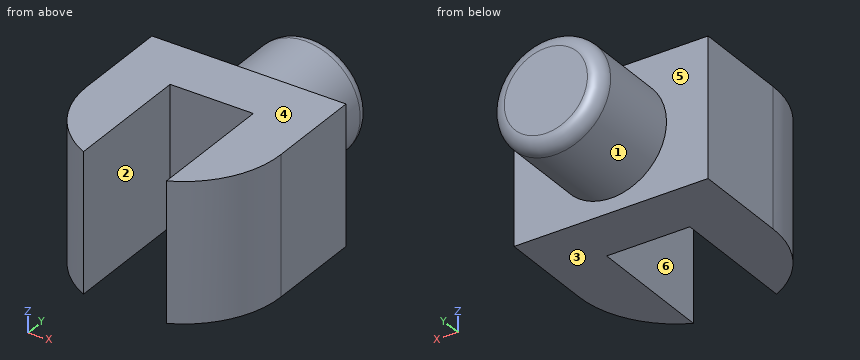
from build123d import *

# Parameters (mm, degrees)
HAND_DEPTH            = 2.5
HAND_DEPTH_BACK       = 2.5
SKETCH3_R             = 2
WRIST_DEPTH           = 7
FINGER_GAP_DEPTH      = 1.5
FINGER_GAP_DEPTH_BACK = 9.215838363
SKETCH2_W             = 3
SKETCH2_H             = 6
EASY_INSERT_R         = 0.5
SCALE1_SCALE          = 2


with BuildPart() as part:
    # Sketch1 → Hand (new, two sides: drawn at the far end of the back side and taken through both)
    with BuildSketch(Plane.XY.offset(-HAND_DEPTH_BACK)):
        with BuildLine():
            Line((-3.5, 0), (-3.5, 3.5))
            Line((-3.5, 3.5), (3.5, 3.5))
            Line((3.5, 3.5), (3.5, 0))
            ThreePointArc((3.5, 0), (0, -3.5), (-3.5, 0))
        make_face()
    extrude(amount=HAND_DEPTH + HAND_DEPTH_BACK)

    # Sketch3 → Wrist (add)
    with BuildSketch(Plane(origin=(0, 0, 0), x_dir=(1, 0, 0), z_dir=(0, 1, 0))):
        with Locations(Location((0, 0, 0), (0, 0, 270))):
            Circle(SKETCH3_R)
    extrude(amount=WRIST_DEPTH)

    # Sketch2 → Finger gap (cut, two sides: drawn at the far end of the back side and taken through both)
    with BuildSketch(Plane(origin=(0, 0, 0), x_dir=(1, 0, 0), z_dir=(0, 1, 0)).offset(-FINGER_GAP_DEPTH_BACK)):
        Rectangle(SKETCH2_W, SKETCH2_H)
    extrude(amount=FINGER_GAP_DEPTH + FINGER_GAP_DEPTH_BACK, mode=Mode.SUBTRACT)

    # Easy insert
    easy_insert_edges = [part.edges().sort_by_distance(p)[0] for p in [
        (0, 7, -2),
    ]]
    fillet(easy_insert_edges, radius=EASY_INSERT_R)


with BuildPart() as part_1:
    # Scale1: scaled about (0, 1.946660074, 0)
    add(part.part.scale(SCALE1_SCALE).moved(Location((0, -1.946660074, 0))))


solid = part_1.part
Read the model definition and answer for the solid it produces. Units are mm, in the model's axes. Face numbers are marked on the shaded views. A direction names the side the tool comes from. Round coordinates to 2 decimals unless told otherwise and drop trailing zeros. Write each loop counter-clockwise with the first axis right and the second up, starting at its lowest first coordinate (ties: lowest second). Pieces come first, ordered by that corner, then holes. Notation, with made-up numbers: M 82.25,-24 L 106.25,-24 A30 ccw 106.25,2 Z; hole C 36.25,40.25 d8. An arc over 180 degrees is marked long. Use a Markdown table: item, result.
1) Straight lines are drawn through the part: line 1 along X through (y, z) = (-1.75, 1.25); line 2 along Y through (x, z) = (2, -2); line 3 along X through (y, z) = (-4.5, -0.25). For each, find the intervals that lie inside material, in ascending order. Write a range as [from, to].
Answers follow:
| item | result |
|---|---|
| line 1 | x = [-7, -3], [3, 7] |
| line 2 | y = [1.05, 12.05] |
| line 3 | x = [-6.52, -3], [3, 6.52] |
2) The part is cut by section A-A (y = -0.5). Write down the section's boundary in (x, z), plus the area to 3 significant figures.
Answers follow:
| item | result |
|---|---|
| outline | M -7,-5 L -3,-5 L -3,5 L -7,5 Z; M 3,-5 L 7,-5 L 7,5 L 3,5 Z |
| area | 80.0 mm2 |
3) The part is cut by section C-C (z = 4.25). Write down the section's boundary in (x, y), plus the area to 3 significant figures.
Answers follow:
| item | result |
|---|---|
| outline | M -7,-1.95 A7 ccw -3,-8.27 L -3,1.05 L 3,1.05 L 3,-8.27 A7 ccw 7,-1.95 L 7,5.05 L -7,5.05 Z |
| area | 116 mm2 |
4) The part is cut by section B-B (x = 0). Write down the section's boundary in (y, z).
Answers follow:
| item | result |
|---|---|
| outline | M 1.05,-5 L 5.05,-5 L 5.05,-4 L 11.05,-4 A1 ccw 12.05,-3 L 12.05,3 A1 ccw 11.05,4 L 5.05,4 L 5.05,5 L 1.05,5 Z |
5) A tool of negligible diameter and unlimited length cuts with its end or side. For the marked faces 4, 5 and 6, from which of +Z, -Z, +X, -X, +Y, -Y can it reach the whole face along a straight path? Write none if from no direction.
Answers follow:
| item | result |
|---|---|
| face 4 | +Z, +X, -X, +Y, -Y |
| face 5 | +Y |
| face 6 | +Z, -Z, -Y |
6) The part is cut by section D-D (y = 10.5). Write down the section's boundary in (x, z), plus the area to 3 significant figures.
Answers follow:
| item | result |
|---|---|
| outline | C 0,0 d8 |
| area | 50.3 mm2 |
7) Flat-ended cylindrical pins translate along their axes: pin 1 (4 mm diameter, centred on x = 4.5, z = 3, fed in from +Y); pin 2 (2 mm diameter, centred on x = -3, y = 8, fed in from +Z). Find the tip coordinate at first contact, or state that the pin passes through.
Answers follow:
| item | result |
|---|---|
| pin 1 | stops at y = 11.97 |
| pin 2 | stops at z = 3.46 |
8) For a pull along X with two mould halves and no side action, classify the marked faces 1, 2 and 3 as pulls with the +X half, pulls with the -X half, needs draft (parallel to the pull), parting line crosses it, or undercut.
Answers follow:
| item | result |
|---|---|
| face 1 | parting line crosses it |
| face 2 | undercut |
| face 3 | needs draft |
